```python
from build123d import *

# Parameters (mm, degrees)
SKETCH1_W                        = 82.55
SKETCH1_H                        = 25.4
BOSS_EXTRUDE1_DEPTH              = 6.35
F_1_4_20_TAPPED_HOLE1_AT_2_COUNT = 2
F_1_4_20_TAPPED_HOLE1_AT_2_PITCH = 38.1


with BuildPart() as part:
    # Sketch1 → Boss-Extrude1 (new body)
    with BuildSketch(Plane.XY):
        with Locations((41.275, 12.7)):
            Rectangle(SKETCH1_W, SKETCH1_H)
    extrude(amount=-BOSS_EXTRUDE1_DEPTH)

    # Sketch3 → 1/4-20 Tapped Hole1 (revolve, cut)
    with BuildSketch(Plane(origin=(22.225, 17.4625, 0), x_dir=(0, -1, 0), z_dir=(1, 0, 0))):
        Polygon((0, 0), (0, 6.35), (6.7437, 6.35), (2.5527, 1.528806005), (2.5527, 0), align=None)
    f_1_4_20_tapped_hole1 = revolve(axis=Axis((22.225, 17.4625, 6.35), (0, 0, -1)), mode=Mode.SUBTRACT)

    # 1/4-20 Tapped Hole1 at 2: 1/4-20 Tapped Hole1 ×2
    with Locations(*[(i * F_1_4_20_TAPPED_HOLE1_AT_2_PITCH, 0, 0) for i in range(1, F_1_4_20_TAPPED_HOLE1_AT_2_COUNT)]):
        add(f_1_4_20_tapped_hole1, mode=Mode.SUBTRACT)


solid = part.part
```
Geometry check sheet. Reference: the model listing, model coordinates, mm. Round coordinates to 2 decimals unless told otherwise and drop trailing zeros. Write item = value, one per line. Start each with the question number.
1. Depth check by flat-ended pin: pin 1 (3 mm diameter, centred on x = 22.22, y = 17.46, fed in from -Z). Enter the tip coordinate at first touch or a pass-through.
2. Mould release check, pull along Y, two halves, no side actions. Record for faces 1 (the face through (24.67, 16.19, -1.76)), 2 (the face through (41, 25.4, -3)), 3 (the face through (41, 13, -6.35)): released by +Y, released by -Y, zero draft, split by the parting line, or undercut.
3. Thickness scan on line 1 (X direction, y = 15.25, z = -3.5); line 2 (X direction, y = 18.75, z = -5.5); line 3 (Y direction, x = 59, z = -0.25). Record the ranges inside material, lowest first.
4. Section check A-A on z = -3.25. Give the number of separate pieces and of enclosed holes in the cut face, then the cut area to 3 significant figures.
Working result:
q1.pin_1 = through
q2.face_1 = undercut
q2.face_2 = released by +Y
q2.face_3 = zero draft
q3.line_1 = 0 to 18.58, 25.87 to 56.68, 63.97 to 82.55
q3.line_2 = 0 to 16.36, 28.09 to 54.46, 66.19 to 82.55
q3.line_3 = 0 to 15.28, 19.64 to 25.4
q4.separate_pieces = 1
q4.enclosed_holes = 2
q4.area = 1,990 mm^2
